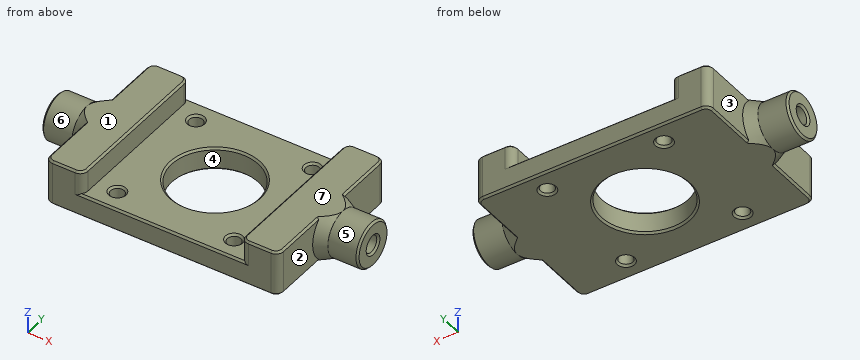
```python
from build123d import *

# Parameters (mm, degrees)
AUFSATZ_LINEAR_AUSTRAGEN1_DEPTH = 6
SKIZZE2_W                       = 10
SKIZZE2_H                       = 42
AUFSATZ_LINEAR_AUSTRAGEN2_DEPTH = 6
SKIZZE3_R                       = 6
AUFSATZ_LINEAR_AUSTRAGEN3_DEPTH = 11
SKIZZE5_R                       = 2.2
SCHNITT_LINEAR_AUSTRAGEN2_DEPTH = 10
SKIZZE4_R                       = 11.5
SKIZZE4_R_2                     = 1.8
SCHNITT_LINEAR_AUSTRAGEN1_DEPTH = 8
FASE1_SIZE                      = 1.5
FASE1_SIZE_2                    = 3
FASE2_SIZE                      = 1.5
FASE2_SIZE_2                    = 3
VERRUNDUNG1_R                   = 2
FASE3_SIZE                      = 0.5


with BuildPart() as part:
    # Skizze1 → Aufsatz-Linear austragen1 (new body)
    with BuildSketch(Plane.XY):
        Polygon((21, 21), (31, 21), (31, -21), (21, -21), (-21, -21), (-31, -21), (-31, 21), (-21, 21), align=None)
    extrude(amount=AUFSATZ_LINEAR_AUSTRAGEN1_DEPTH)

    # Skizze2 → Aufsatz-Linear austragen2 (add)
    with BuildSketch(Plane.XY.offset(6)):
        with Locations((26, 0)):
            Rectangle(SKIZZE2_W, SKIZZE2_H)
        with Locations((-26, 0)):
            Rectangle(SKIZZE2_W, SKIZZE2_H)
    extrude(amount=AUFSATZ_LINEAR_AUSTRAGEN2_DEPTH)

    # Skizze3 → Aufsatz-Linear austragen3 (add)
    with BuildSketch(Plane(origin=(31, 0, 0), x_dir=(0, 0, -1), z_dir=(1, 0, 0))):
        with Locations((-6, 0)):
            Circle(SKIZZE3_R)
    aufsatz_linear_austragen3 = extrude(amount=AUFSATZ_LINEAR_AUSTRAGEN3_DEPTH)

    # Skizze5 → Schnitt-Linear austragen2 (cut)
    with BuildSketch(Plane(origin=(42, 0, 0), x_dir=(0, 0, -1), z_dir=(1, 0, 0))):
        with Locations(Location((-6, 0, 0), (0, 0, 90))):
            Circle(SKIZZE5_R)
    schnitt_linear_austragen2 = extrude(amount=-SCHNITT_LINEAR_AUSTRAGEN2_DEPTH, mode=Mode.SUBTRACT)

    # Spiegeln1: Aufsatz-Linear austragen3, Schnitt-Linear austragen2 across plane
    add(aufsatz_linear_austragen3.mirror(Plane(origin=(0, 0, 0), x_dir=(0, 0, 1), z_dir=(1, 0, 0))))
    add(schnitt_linear_austragen2.mirror(Plane(origin=(0, 0, 0), x_dir=(0, 0, 1), z_dir=(1, 0, 0))), mode=Mode.SUBTRACT)

    # Skizze4 → Schnitt-Linear austragen1 (cut)
    with BuildSketch(Plane.XY.offset(6)):
        Circle(SKIZZE4_R)
        with Locations((-15.5, 15.5)):
            Circle(SKIZZE4_R_2)
        with Locations((15.5, 15.5)):
            Circle(SKIZZE4_R_2)
        with Locations((15.5, -15.5)):
            Circle(SKIZZE4_R_2)
        with Locations((-15.5, -15.5)):
            Circle(SKIZZE4_R_2)
    extrude(amount=-SCHNITT_LINEAR_AUSTRAGEN1_DEPTH, mode=Mode.SUBTRACT)

    # Fase1
    # the kernel refuses this chamfer: 3, 1.5 mm, written as the material it adds along each edge
    with BuildSketch(Plane(origin=(31, 0, 6), x_dir=(0, 0, -1), z_dir=(0, -1, 0))) as fase1_piece_1_section:
        Polygon((6 + FASE1_SIZE, 0), (6, FASE1_SIZE_2), (6, 0), align=None)
    fase1_piece_1 = revolve(axis=Axis((31, 0, 6), (1, 0, 0)), revolution_arc=179.999999686, mode=Mode.PRIVATE)
    fase1_piece_1 = split(fase1_piece_1, bisect_by=Plane(origin=(32.485350769, 6.720701537, 0), z_dir=(0, 0, 1)), keep=Keep.TOP, mode=Mode.PRIVATE)
    fase1_piece_1 = split(fase1_piece_1, bisect_by=Plane(origin=(32.485350769, 6.720701537, 12), z_dir=(0, 0, -1)), keep=Keep.TOP, mode=Mode.PRIVATE)
    add(fase1_piece_1)
    with BuildSketch(Plane(origin=(31, 0, 6), x_dir=(0, 5.472961761905791e-09, 1.0), z_dir=(0, 1.0, -5.472961761905791e-09))) as fase1_piece_2_section:
        Polygon((6 + FASE1_SIZE, 0), (6, FASE1_SIZE_2), (6, 0), align=None)
    fase1_piece_2 = revolve(axis=Axis((31, 0, 6), (1, 0, 0)), revolution_arc=180.000000314, mode=Mode.PRIVATE)
    fase1_piece_2 = split(fase1_piece_2, bisect_by=Plane(origin=(32.485350772, -6.720701535, 0), z_dir=(0, 0, 1)), keep=Keep.TOP, mode=Mode.PRIVATE)
    fase1_piece_2 = split(fase1_piece_2, bisect_by=Plane(origin=(32.485350772, -6.720701535, 12), z_dir=(0, 0, -1)), keep=Keep.TOP, mode=Mode.PRIVATE)
    add(fase1_piece_2)

    # Fase2
    # the kernel refuses this chamfer: 3, 1.5 mm, written as the material it adds along each edge
    with BuildSketch(Plane(origin=(-31, 0, 6), x_dir=(0, 0, -1), z_dir=(0, -1, 0))) as fase2_piece_1_section:
        Polygon((6 + FASE2_SIZE, 0), (6, -FASE2_SIZE_2), (6, 0), align=None)
    fase2_piece_1 = revolve(axis=Axis((-31, 0, 6), (1, 0, 0)), revolution_arc=179.999999686, mode=Mode.PRIVATE)
    fase2_piece_1 = split(fase2_piece_1, bisect_by=Plane(origin=(-32.485350769, 6.720701537, 0), z_dir=(0, 0, 1)), keep=Keep.TOP, mode=Mode.PRIVATE)
    fase2_piece_1 = split(fase2_piece_1, bisect_by=Plane(origin=(-32.485350769, 6.720701537, 12), z_dir=(0, 0, -1)), keep=Keep.TOP, mode=Mode.PRIVATE)
    add(fase2_piece_1)
    with BuildSketch(Plane(origin=(-31, 0, 6), x_dir=(0, 5.472961761905791e-09, 1.0), z_dir=(0, 1.0, -5.472961761905791e-09))) as fase2_piece_2_section:
        Polygon((6 + FASE2_SIZE, 0), (6, -FASE2_SIZE_2), (6, 0), align=None)
    fase2_piece_2 = revolve(axis=Axis((-31, 0, 6), (1, 0, 0)), revolution_arc=180.000000314, mode=Mode.PRIVATE)
    fase2_piece_2 = split(fase2_piece_2, bisect_by=Plane(origin=(-32.485350772, -6.720701535, 0), z_dir=(0, 0, 1)), keep=Keep.TOP, mode=Mode.PRIVATE)
    fase2_piece_2 = split(fase2_piece_2, bisect_by=Plane(origin=(-32.485350772, -6.720701535, 12), z_dir=(0, 0, -1)), keep=Keep.TOP, mode=Mode.PRIVATE)
    add(fase2_piece_2)

    # Verrundung1
    verrundung1_edges = [part.edges().sort_by_distance(p)[0] for p in [
        (31, 21, 6),
        (31, -21, 6),
        (-31, -21, 6),
        (-31, 21, 6),
        (21, -21, 9),
        (21, 21, 9),
        (-21, 21, 9),
        (-21, -21, 9),
    ]]
    fillet(verrundung1_edges, radius=VERRUNDUNG1_R)

    # Fase3
    fase3_edges = [part.edges().sort_by_distance(p)[0] for p in [
        (-31, -11.75, 0),
        (-31, 11.75, 12),
        (-21, 0, 12),
        (0, -21, 0),
        (26, -21, 12),
        (-26, -21, 12),
        (-26, 21, 12),
        (-31, -11.75, 12),
        (-30.414213562, 20.414213562, 12),
        (-30.414213562, -20.414213562, 12),
        (-21.585786438, 20.414213562, 12),
        (-21.585786438, -20.414213562, 12),
        (21, 0, 12),
        (31, 11.75, 12),
        (26, 21, 12),
        (30.414213562, 20.414213562, 12),
        (30.414213562, -20.414213562, 12),
        (21.585786438, 20.414213562, 12),
        (21.585786438, -20.414213562, 12),
        (0, 21, 0),
        (-31, 11.75, 0),
        (31, -11.75, 0),
        (30.414213562, 20.414213562, 0),
        (-30.414213562, 20.414213562, 0),
        (30.414213562, -20.414213562, 0),
        (-30.414213562, -20.414213562, 0),
        (0, 21, 6),
        (0, -21, 6),
        (42, 0, 12),
        (42, -2.2, 6),
        (-42, 0, 12),
        (-42, -2.2, 6),
        (-17.3, -15.5, 0),
        (-17.3, -15.5, 6),
        (13.7, -15.5, 0),
        (13.7, -15.5, 6),
        (13.7, 15.5, 0),
        (13.7, 15.5, 6),
        (-17.3, 15.5, 0),
        (-17.3, 15.5, 6),
        (-11.5, 0, 0),
        (-11.5, 0, 6),
        (31, -11.75, 12),
        (31, 11.75, 0),
    ]]
    chamfer(fase3_edges, length=FASE3_SIZE)


solid = part.part
```
For this review, take the finished solid that the model builds, in its own axes (mm). Face numbers are marked on the shaded views. A direction names the side the tool comes from. Give positions to 0.01 mm unless a question says otherwise; leave off trailing zeros. Loops run counter-clockwise (first coordinate to the right, second up) from the corner with the lowest first, then second, coordinate; pieces in that order, holes last. Notation, with made-up numbers: M 83.5,11 L 87.5,11 A27 ccw 87.5,32 Z; hole C 27.25,-5.5 d11. An arc over 180 degrees is marked long. One line per item, written item: value. Start each with the question number.
Q1. Add section A-A (y = 15.5). Count the separate pieces of the cut face and the enclosed holes in it, and give its area (3 significant figures).
Q2. Machinability: for the marked faces 5, 6 and 7, which of the approach directions +Z, -Z, +X, -X, +Y, -Y give a long, thin tool a straight path to every point of the face, cutting with its end or side? Answer none if there is none.
Q3. Add section C-C (x = 15.5). Give the boundary of the cut face in (y, z), and give its area (3 significant figures).
Q4. Draft analysis for pull direction X (two halves, no side actions). For the marked faces 1, 2, 3 and 4, state which applies: released by +X, released by -X, zero draft, split by the parting line, or undercut.
Q5. For L1, parallel to Y at x = -15.5, z = 3.6; L2, parallel to X at y = 14.5, z = 4.25; L3, parallel to X at y = -14, z = 5, list the stretches that pass through material, from the lowest coordinate up.
Q6. Clearance check with flat-ended pins moving along their axes: pin 1 Ø1 at (x, z) = (-33.5, 10) entering from +Y; pin 2 Ø5.5 at (y, z) = (13.5, 5.5) entering from +X; pin 3 Ø3.5 at (y, z) = (0, 6.5) entering from +X. State where each tip first meets the part, or that it passes through.
Q7. Add section B-B (x = 0). Give the boundary of the cut face in (y, z).
Reply:
1. separate pieces: 3
1. enclosed holes: 0
1. area: 447 mm²
2. face 5: +X
2. face 6: -X
2. face 7: +Z, +X, -X, +Y, -Y
3. outline: M -21,0.5 L -20.5,0 L -17.8,0 L -17.3,0.5 L -17.3,5.5 L -17.8,6 L -20.5,6 L -21,5.5 Z; M -13.7,0.5 L -13.2,0 L 13.2,0 L 13.7,0.5 L 13.7,5.5 L 13.2,6 L -13.2,6 L -13.7,5.5 Z; M 17.3,0.5 L 17.8,0 L 20.5,0 L 21,0.5 L 21,5.5 L 20.5,6 L 17.8,6 L 17.3,5.5 Z
3. area: 207 mm²
4. face 1: zero draft
4. face 2: released by +X
4. face 3: released by -X
4. face 4: undercut
5. L1: -21 to -17.3, -13.7 to 13.7, 17.3 to 21
5. L2: -31 to -17, -14 to 14, 17 to 31
5. L3: -31 to -16.49, -14.51 to 14.51, 16.49 to 31
6. pin 1: y = 5.29
6. pin 2: x = 31
6. pin 3: x = 41.55
7. outline: M -21,0.5 L -20.5,0 L -12,0 L -11.5,0.5 L -11.5,5.5 L -12,6 L -20.5,6 L -21,5.5 Z; M 11.5,0.5 L 12,0 L 20.5,0 L 21,0.5 L 21,5.5 L 20.5,6 L 12,6 L 11.5,5.5 Z
